CAD build for the part. Positions are in the model's coordinates, mm. Face numbers are marked on the shaded views. A direction names the side the tool comes from. Round coordinates to 2 decimals unless told otherwise and drop trailing zeros. Loops run counter-clockwise (first coordinate to the right, second up) from the corner with the lowest first, then second, coordinate; pieces in that order, holes last. Notation, with made-up numbers: M 38,53 L 76,53 A13 cw 76,74 Z; hole C -17.75,-13 d8. An arc over 180 degrees is marked long. Use one line per item in the form item = value.
from build123d import *

# Parameters (mm, degrees)
BOSS_EXTRUDE1_DEPTH = 27.5
CUT_EXTRUDE1_REACH  = 72.266
CUT_EXTRUDE2_REACH  = 71.98
BOSS_EXTRUDE2_DEPTH = 5
BOSS_EXTRUDE3_START = -55
BOSS_EXTRUDE3_DEPTH = 5


with BuildPart() as part:
    # Sketch1 → Boss-Extrude1 (new, symmetric)
    with BuildSketch(Plane(origin=(0, 0, 0), x_dir=(0, 0, -1), z_dir=(1, 0, 0))):
        Polygon((0, 0), (50, 0), (50, 45), (46, 45), (46, 4), (0, 4), align=None)
    extrude(amount=BOSS_EXTRUDE1_DEPTH, both=True)

    # Sketch2 → Cut-Extrude1 (cut, up to next)
    with BuildSketch(Plane(origin=(0, 4, 0), x_dir=(1, 0, 0), z_dir=(0, 1, 0)), mode=Mode.PRIVATE) as cut_extrude1_sk1:
        with BuildLine():
            Line((-12.9, 9.1), (-12.9, 38.9))
            ThreePointArc((-12.9, 38.9), (-15, 41), (-17.1, 38.9))
            Line((-17.1, 38.9), (-17.1, 9.1))
            ThreePointArc((-17.1, 9.1), (-16.48492424, 7.61507576), (-15, 7))
            ThreePointArc((-15, 7), (-13.51507576, 7.61507576), (-12.9, 9.1))
        make_face()
    cut_extrude1_tool1 = extrude(cut_extrude1_sk1.sketch, amount=-CUT_EXTRUDE1_REACH, mode=Mode.PRIVATE) & part.part
    # Sketch2 → Cut-Extrude1 (cut, up to next)
    with BuildSketch(Plane(origin=(0, 4, 0), x_dir=(1, 0, 0), z_dir=(0, 1, 0)), mode=Mode.PRIVATE) as cut_extrude1_sk2:
        with BuildLine():
            Line((12.9, 38.9), (12.9, 9.1))
            ThreePointArc((12.9, 9.1), (13.51507576, 7.61507576), (15, 7))
            ThreePointArc((15, 7), (16.48492424, 7.61507576), (17.1, 9.1))
            Line((17.1, 9.1), (17.1, 38.9))
            ThreePointArc((17.1, 38.9), (15, 41), (12.9, 38.9))
        make_face()
    cut_extrude1_tool2 = extrude(cut_extrude1_sk2.sketch, amount=-CUT_EXTRUDE1_REACH, mode=Mode.PRIVATE) & part.part
    add(cut_extrude1_tool1.solids().sort_by_distance((-15, 4, -24))[0], mode=Mode.SUBTRACT)
    add(cut_extrude1_tool2.solids().sort_by_distance((15, 4, -24))[0], mode=Mode.SUBTRACT)

    # Sketch3 → Cut-Extrude2 (cut, up to next)
    with BuildSketch(Plane.XY.offset(-46), mode=Mode.PRIVATE) as cut_extrude2_sk1:
        with BuildLine():
            ThreePointArc((11, 26.216818276), (0, 37.216818276), (-11, 26.216818276))
            ThreePointArc((-11, 26.216818276), (0, 15.216818276), (11, 26.216818276))
        make_face()
    cut_extrude2_tool1 = extrude(cut_extrude2_sk1.sketch, amount=-CUT_EXTRUDE2_REACH, mode=Mode.PRIVATE) & part.part
    # Sketch3 → Cut-Extrude2 (cut, up to next)
    with BuildSketch(Plane.XY.offset(-46), mode=Mode.PRIVATE) as cut_extrude2_sk2:
        with BuildLine():
            ThreePointArc((-17.2, 10.716818276), (-15.5, 9.016818276), (-13.8, 10.716818276))
            ThreePointArc((-13.8, 10.716818276), (-15.5, 12.416818276), (-17.2, 10.716818276))
        make_face()
    cut_extrude2_tool2 = extrude(cut_extrude2_sk2.sketch, amount=-CUT_EXTRUDE2_REACH, mode=Mode.PRIVATE) & part.part
    # Sketch3 → Cut-Extrude2 (cut, up to next)
    with BuildSketch(Plane.XY.offset(-46), mode=Mode.PRIVATE) as cut_extrude2_sk3:
        with BuildLine():
            ThreePointArc((-17.2, 41.716818276), (-15.5, 40.016818276), (-13.8, 41.716818276))
            ThreePointArc((-13.8, 41.716818276), (-15.5, 43.416818276), (-17.2, 41.716818276))
        make_face()
    cut_extrude2_tool3 = extrude(cut_extrude2_sk3.sketch, amount=-CUT_EXTRUDE2_REACH, mode=Mode.PRIVATE) & part.part
    # Sketch3 → Cut-Extrude2 (cut, up to next)
    with BuildSketch(Plane.XY.offset(-46), mode=Mode.PRIVATE) as cut_extrude2_sk4:
        with BuildLine():
            ThreePointArc((13.8, 41.716818276), (15.5, 40.016818276), (17.2, 41.716818276))
            ThreePointArc((17.2, 41.716818276), (15.5, 43.416818276), (13.8, 41.716818276))
        make_face()
    cut_extrude2_tool4 = extrude(cut_extrude2_sk4.sketch, amount=-CUT_EXTRUDE2_REACH, mode=Mode.PRIVATE) & part.part
    # Sketch3 → Cut-Extrude2 (cut, up to next)
    with BuildSketch(Plane.XY.offset(-46), mode=Mode.PRIVATE) as cut_extrude2_sk5:
        with BuildLine():
            ThreePointArc((17.2, 10.716818276), (15.5, 12.416818276), (13.8, 10.716818276))
            ThreePointArc((13.8, 10.716818276), (15.5, 9.016818276), (17.2, 10.716818276))
        make_face()
    cut_extrude2_tool5 = extrude(cut_extrude2_sk5.sketch, amount=-CUT_EXTRUDE2_REACH, mode=Mode.PRIVATE) & part.part
    add(cut_extrude2_tool1.solids().sort_by_distance((0, 26.216818, -46))[0], mode=Mode.SUBTRACT)
    add(cut_extrude2_tool2.solids().sort_by_distance((-15.5, 10.716818, -46))[0], mode=Mode.SUBTRACT)
    add(cut_extrude2_tool3.solids().sort_by_distance((-15.5, 41.716818, -46))[0], mode=Mode.SUBTRACT)
    add(cut_extrude2_tool4.solids().sort_by_distance((15.5, 41.716818, -46))[0], mode=Mode.SUBTRACT)
    add(cut_extrude2_tool5.solids().sort_by_distance((15.5, 10.716818, -46))[0], mode=Mode.SUBTRACT)

    # Sketch5 → Boss-Extrude2 (add)
    with BuildSketch(Plane(origin=(27.5, 0, 0), x_dir=(0, 0, -1), z_dir=(1, 0, 0))):
        Polygon((46, 24.5), (23, 4), (46, 4), align=None)
    extrude(amount=-BOSS_EXTRUDE2_DEPTH)

    # Sketch5<2> → Boss-Extrude3 (add)
    with BuildSketch(Plane(origin=(27.5, 0, 0), x_dir=(0, 0, -1), z_dir=(1, 0, 0)).offset(BOSS_EXTRUDE3_START)):
        Polygon((46, 24.5), (23, 4), (46, 4), align=None)
    extrude(amount=BOSS_EXTRUDE3_DEPTH)


solid = part.part
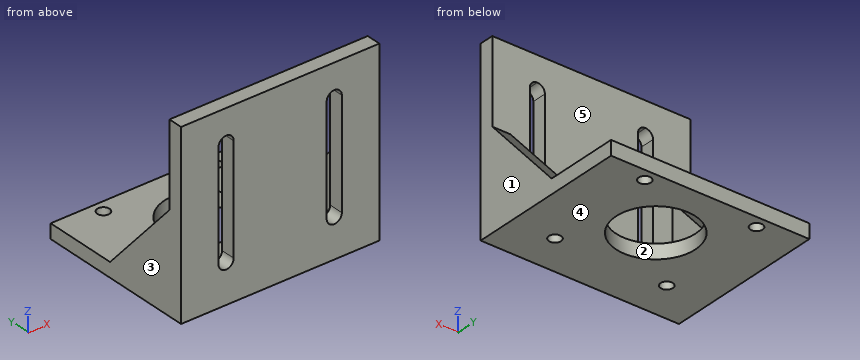
1. Cut at C-C on y = 22. Write the cut outline in (x, z), and give its area (3 significant figures).
Completed:
outline = M -27.5,-50 L -10.16,-50 L -10.16,-46 L -22.5,-46 L -22.5,-43.2 L -27.5,-43.2 Z; M 10.16,-50 L 27.5,-50 L 27.5,-43.2 L 22.5,-43.2 L 22.5,-46 L 10.16,-46 Z
area = 167 mm2
2. Drop flat-ended pins along their axis: P1, Ø8, axis at x = 20.5, y = 22, coming from the +Z side; P2, Ø3, axis at x = 18.5, z = -42.5, coming from the +Y side; P3, Ø5, axis at x = -19, y = 28.5, coming from the +Z side. Give the stop position or say it passes through.
Completed:
P1 = -39.31
P2 = 4
P3 = -46
3. Tool access for the marked faces 4 and 5: list every direction of +Z, -Z, +X, -X, +Y, -Y with a clear straight run to the whole face (end or side of a thin tool).
Completed:
face_4 = -Z, +X, -X, +Y, -Y
face_5 = +Z, +Y
4. Cut at A-A on z = -22. Write the cut outline in (x, y), and give its area (3 significant figures).
Completed:
outline = M -27.5,0 L -17.1,0 L -17.1,4 L -27.5,4 Z; M -12.9,0 L 12.9,0 L 12.9,4 L -12.9,4 Z; M 17.1,0 L 27.5,0 L 27.5,4 L 17.1,4 Z
area = 186 mm2
5. Cut at D-D on x = 21. Write the cut outline in (y, z).
Completed:
outline = M 0,-50 L 45,-50 L 45,-46 L 4,-46 L 4,0 L 0,0 Z
6. Pull direction X, two halves, no side cores. Call the marked faces 1, 2 and 3: +X half, -X half, draft (parallel to the pull), parting line (faces both ways), or undercut.
Completed:
face_1 = +X half
face_2 = undercut
face_3 = -X half
7. Cut at B-B on x = 0. Write the cut outline in (y, z).
Completed:
outline = M 0,-50 L 15.22,-50 L 15.22,-46 L 4,-46 L 4,0 L 0,0 Z; M 37.22,-50 L 45,-50 L 45,-46 L 37.22,-46 Z
8. Probe line 1 along Y through (x, z) = (-15.5, -48.9); line 2 along Y through (x, z) = (0, -49.05); line 3 along Y through (x, z) = (5, -30). List the from-to ranges inside material, lowest first. Write a range as from..to.
Completed:
line_1 = 0..9.02, 12.42..40.02, 43.42..45
line_2 = 0..15.22, 37.22..45
line_3 = 0..4
